For this review, take the finished solid that the model builds, in its own axes (mm). Coordinates: 2 decimals unless noted, no trailing zeros. Write each loop counter-clockwise with the first axis right and the second up, starting at its lowest first coordinate (ties: lowest second). Pieces come first, ordered by that corner, then holes. Notation, with made-up numbers: (87, -16) - (130, -16) arc R22 ccw to (130, 8) - close; hole circle Ø6 at (-21, 1.25). An arc over 180 degrees is marked (long way). Use one line per item in the form item = value. Start each with the question number.
1) We need section A-A (z = -169). Give the boundary of the cut face in (x, y), plus the area to 3 significant figures.
2) For L1, parallel to Z at x = -15.35, y = 3 (3 decimals); L2, parallel to Y at x = -14, z = -644; L3, parallel to Y at x = -14.8, z = -644.4 (3 decimals), list the stretches that pass through material, from the lowest coordinate up. Write a range as from..to.
3) We need section B-B (x = -6). Give the boundary of the cut face in (y, z), plus the area to 3 significant figures.
4) Insertion check: P1, Ø3, axis at x = 0, z = -442, coming from the +Y side; P2, Ø5, axis at y = 3, z = -16, coming from the -X side. Each pin has a flat end and moves straight along its axis. Give the tip position at first contact, or say it passes through.
Autodesk Inventor part; units mm, degrees
ref_plane "YZ Plane" through (0, 0, 0) normal (1, 0, 0) x (0, 1, 0)
ref_plane "XZ Plane" through (0, 0, 0) normal (0, 1, 0) x (-1, 0, 0)
ref_plane "XY Plane" through (0, 0, 0) normal (0, 0, 1) x (1, 0, 0)
sketch "Sketch1" plane through (0, 0, 0) normal (0, 0, 1) x (1, 0, 0)
  line L0 (-16, 12.5) -> (-13, 12.5)
  line L1 (-13, 12.5) -> (-13, -9.5)
  line L2 (-13, -9.5) -> (13, -9.5)
  line L3 (13, -9.5) -> (13, 12.5)
  line L4 (13, 12.5) -> (16, 12.5)
  line L5 (16, 12.5) -> (16, -12.5)
  line L6 (16, -12.5) -> (-16, -12.5)
  line L7 (-16, -12.5) -> (-16, 12.5)
  point P0 (0, 0)
  dimension "d0" = 3
  dimension "d2" = 3
  dimension "d3" = 25
  dimension "d4" = 32
  dimension "d5" = 16
  dimension "d7" = 12.5
  dimension "d8" = 3
  dimension "d74" = 25
extrude "Extrusion1" add sketch "Sketch1" against normal blind 660.4
sketch "Sketch6" plane through (-16, -12.5, 0) normal (-1, 0, 0) x (0, 0, 1)
  circle A0 centre (-37.4708, 12.3) radius 3.175
  circle A1 centre (-177.8, 12.3) radius 3.175
  circle A2 centre (-340.3166, 12.3) radius 3.175
  circle A3 centre (-644.4, 15.5) radius 3.175
  line L0 (0, 25) -> (-660.4, 25)
  line L1 (0, 3) -> (-660.4, 3)
  line L2 (-660.4, 0) -> (-660.4, 25)
  circle A4 centre (-16, 15.5) radius 3.175
  line L3 (0, 0) -> (0, 25)
  point P0 (0, 12.5)
  dimension "d89" = 6.35
  dimension "d92" = 16
  dimension "d93" = 6.35
  dimension "d94" = 16
  dimension "d103" = 12.5
hole "Hole3" at (-16, 3, -644.4) at (-16, 3, -16) direction (1, 0, 0) diameter 6.35 depth 3 tip angle 118
equation "\"d2\" = d0"
equation "\"d8\" = d0"
equation "\"d74\" = d3"
properties part number "26in C-Channel Right" material "Aluminum 6061"
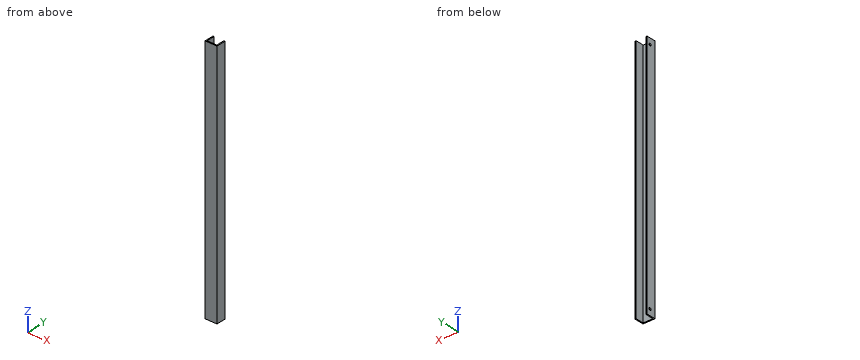
Determined:
q1.outline = (-16, -12.5) - (16, -12.5) - (16, 12.5) - (13, 12.5) - (13, -9.5) - (-13, -9.5) - (-13, 12.5) - (-16, 12.5) - close
q1.area = 228 mm²
q2.L1 = -660.4..-647.575, -641.225..-19.175, -12.825..0
q2.L2 = -12.5..-0.15, 6.15..12.5
q2.L3 = -12.5..-0.175, 6.175..12.5
q3.outline = (-12.5, -660.4) - (-9.5, -660.4) - (-9.5, 0) - (-12.5, 0) - close
q3.area = 1,980 mm²
q4.P1 = -9.5
q4.P2 = 13
